Read the model definition and answer for the solid it produces. Units are mm, in the model's axes. Face numbers are marked on the shaded views. A direction names the side the tool comes from. Coordinates: 2 decimals unless noted, no trailing zeros. Write each loop counter-clockwise with the first axis right and the second up, starting at its lowest first coordinate (ties: lowest second). Pieces come first, ordered by that corner, then holes. Notation, with made-up numbers: M 80.5,-20 L 98.5,-20 A26 cw 98.5,0 Z; hole C -24.5,65 d9. An arc over 180 degrees is marked long. Use a Markdown table: item, result. Add a question column.
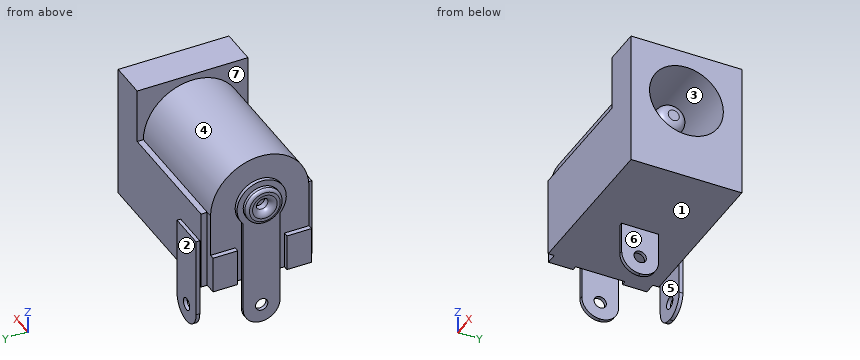
from build123d import *

# Parameters (mm, degrees)
BOSS_EXTRUDE1_DEPTH  = 6.5
BOSS_EXTRUDE2_REACH  = 18.078
SKETCH2_R            = 4
BOSS_EXTRUDE3_DEPTH  = 3
CUT_EXTRUDE1_START   = -0.4
CUT_EXTRUDE1_DEPTH   = 0.4
SKETCH5_W            = 3
SKETCH5_H            = 4
BOSS_EXTRUDE4_DEPTH  = 0.3
SKETCH6_W            = 3
SKETCH6_H            = 0.3
BOSS_EXTRUDE5_DEPTH  = 4
SKETCH7_R            = 0.5
CUT_EXTRUDE4_DEPTH   = 17.01530518
SKETCH8_W            = 6.5
SKETCH8_H            = 0.5
BOSS_EXTRUDE6_DEPTH  = 0.2
BOSS_EXTRUDE7_DEPTH  = 0.3
SKETCH10_W           = 0.3
SKETCH10_H           = 3
BOSS_EXTRUDE8_DEPTH  = 4
SKETCH12_W           = 0.3
SKETCH12_H           = 3
BOSS_EXTRUDE9_DEPTH  = 4
SKETCH11_R           = 0.5
CUT_EXTRUDE5_DEPTH   = 19.364367672
SKETCH13_R           = 3
CUT_EXTRUDE6_DEPTH   = 10
SKETCH14_R           = 1.5
BOSS_EXTRUDE10_DEPTH = 0.5
SKETCH15_R           = 0.5
CUT_EXTRUDE7_DEPTH   = 1
FILLET1_R            = 0.5
FILLET2_R            = 0.25
SKETCH16_R           = 1.2
BOSS_EXTRUDE11_DEPTH = 8
FILLET4_R            = 0.75


with BuildPart() as part:
    # Sketch1 → Boss-Extrude1 (new body)
    with BuildSketch(Plane.XY):
        Polygon((7, 4.5), (-5.873443246, 4.5), (-5.873443246, 4), (-7, 4), (-7, -4), (-5.873443246, -4), (-5.873443246, -4.5), (7, -4.5), align=None)
    extrude(amount=BOSS_EXTRUDE1_DEPTH)

    # Boss-Extrude2: up to this face of the body (flat: up to its plane)
    boss_extrude2_end = Plane(part.part.faces().sort_by_distance((-7, 0, 3.25))[0])
    # Sketch2 → Boss-Extrude2 (add, up to the picked face)
    with BuildSketch(Plane(origin=(7, 0, 0), x_dir=(0, 0, -1), z_dir=(1, 0, 0)), mode=Mode.PRIVATE) as boss_extrude2_sk1:
        with Locations((-6.5, 0)):
            Circle(SKETCH2_R)
    boss_extrude2_tool1 = split(extrude(boss_extrude2_sk1.sketch, amount=-BOSS_EXTRUDE2_REACH, mode=Mode.PRIVATE), bisect_by=boss_extrude2_end, keep=Keep.BOTH, mode=Mode.PRIVATE)
    add(boss_extrude2_tool1.solids().sort_by(Axis((7, 0, 6.5), (-1, 0, 0)))[0])

    # Sketch3 → Boss-Extrude3 (add)
    with BuildSketch(Plane(origin=(7, 0, 0), x_dir=(0, 0, -1), z_dir=(1, 0, 0))):
        with BuildLine():
            Line((-11, -4.5), (-6.5, -4.5))
            Line((-6.5, -4.5), (-6.5, -4))
            ThreePointArc((-6.5, -4), (-10.5, 0), (-6.5, 4))
            Line((-6.5, 4), (-6.5, 4.5))
            Line((-6.5, 4.5), (-11, 4.5))
            Line((-11, 4.5), (-11, 0.782604766))
            Line((-11, 0.782604766), (-11, -4.5))
        make_face()
    extrude(amount=-BOSS_EXTRUDE3_DEPTH)

    # Sketch4 → Cut-Extrude1 (cut)
    with BuildSketch(Plane.ZY.offset(7).offset(CUT_EXTRUDE1_START)):
        with BuildLine():
            Line((3, 4), (3, 2))
            Line((3, 2), (0, 2))
            Line((0, 2), (0, -2))
            Line((0, -2), (3, -2))
            Line((3, -2), (3, -4))
            Line((3, -4), (6.5, -4))
            ThreePointArc((6.5, -4), (10.5, 0), (6.5, 4))
            Line((6.5, 4), (3, 4))
        make_face()
    extrude(amount=CUT_EXTRUDE1_DEPTH, mode=Mode.SUBTRACT)

    # Sketch5 → Boss-Extrude4 (add)
    with BuildSketch(Plane(origin=(0, 4.5, 0), x_dir=(1, 0, 0), z_dir=(0, 1, 0))):
        with Locations((-4.373443246, -2)):
            Rectangle(SKETCH5_W, SKETCH5_H)
    extrude(amount=BOSS_EXTRUDE4_DEPTH)

    # Sketch6 → Boss-Extrude5 (add)
    with BuildSketch(Plane(origin=(0, 0, 0), x_dir=(-1, 0, 0), z_dir=(0, 0, -1))):
        with Locations((4.373443246, 4.65)):
            Rectangle(SKETCH6_W, SKETCH6_H)
    extrude(amount=BOSS_EXTRUDE5_DEPTH)

    # Sketch7 → Cut-Extrude4 (cut, through all)
    with BuildSketch(Plane(origin=(0, 4.8, 0), x_dir=(1, 0, 0), z_dir=(0, 1, 0))):
        with Locations(Location((-4.373443246, 2.5, 0), (0, 0, 270))):
            Circle(SKETCH7_R)
        with BuildLine():
            Line((-5.873443246, 4), (-5.873443246, 2.5))
            ThreePointArc((-5.873443246, 2.5), (-5.434103418, 3.560660172), (-4.373443246, 4))
            Line((-4.373443246, 4), (-5.873443246, 4))
        make_face()
        with BuildLine():
            Line((-2.873443246, 4), (-4.373443246, 4))
            ThreePointArc((-4.373443246, 4), (-3.312783074, 3.560660172), (-2.873443246, 2.5))
            Line((-2.873443246, 2.5), (-2.873443246, 4))
        make_face()
    extrude(amount=-CUT_EXTRUDE4_DEPTH, mode=Mode.SUBTRACT)

    # Sketch8 → Boss-Extrude6 (add)
    with BuildSketch(Plane.ZY.offset(5.873443246)):
        with Locations((3.25, 4.25)):
            Rectangle(SKETCH8_W, SKETCH8_H)
        with Locations((3.25, -4.25)):
            Rectangle(SKETCH8_W, SKETCH8_H)
    extrude(amount=BOSS_EXTRUDE6_DEPTH)

    # Sketch9 → Boss-Extrude7 (add)
    with BuildSketch(Plane.ZY.offset(6.6)):
        with BuildLine():
            Line((5.177124344, 1.5), (0, 1.5))
            Line((0, 1.5), (0, -1.5))
            Line((0, -1.5), (5.177124344, -1.5))
            ThreePointArc((5.177124344, -1.5), (8.5, 0), (5.177124344, 1.5))
        make_face()
    extrude(amount=BOSS_EXTRUDE7_DEPTH)

    # Sketch10 → Boss-Extrude8 (add)
    with BuildSketch(Plane(origin=(0, 0, 0), x_dir=(-1, 0, 0), z_dir=(0, 0, -1))):
        with Locations((6.75, 0)):
            Rectangle(SKETCH10_W, SKETCH10_H)
    extrude(amount=BOSS_EXTRUDE8_DEPTH)

    # Sketch12 → Boss-Extrude9 (add)
    with BuildSketch(Plane(origin=(0, 0, 0), x_dir=(-1, 0, 0), z_dir=(0, 0, -1))):
        with Locations((0.45, 0)):
            Rectangle(SKETCH12_W, SKETCH12_H)
    extrude(amount=BOSS_EXTRUDE9_DEPTH)

    # Sketch11 → Cut-Extrude5 (cut, through all)
    with BuildSketch(Plane.ZY.offset(6.9)):
        with Locations(Location((-2.5, 0, 0), (0, 0, 270))):
            Circle(SKETCH11_R)
        with BuildLine():
            Line((-2.5, 1.5), (-4, 1.5))
            Line((-4, 1.5), (-4, 0))
            ThreePointArc((-4, 0), (-3.560660172, 1.060660172), (-2.5, 1.5))
        make_face()
        with BuildLine():
            ThreePointArc((-2.5, -1.5), (-3.560660172, -1.060660172), (-4, 0))
            Line((-4, 0), (-4, -1.5))
            Line((-4, -1.5), (-2.5, -1.5))
        make_face()
    extrude(amount=-CUT_EXTRUDE5_DEPTH, mode=Mode.SUBTRACT)

    # Sketch13 → Cut-Extrude6 (cut)
    with BuildSketch(Plane(origin=(7, 0, 0), x_dir=(0, 0, -1), z_dir=(1, 0, 0))):
        with Locations(Location((-6.7, 0, 0), (0, 0, 90))):
            Circle(SKETCH13_R)
    extrude(amount=-CUT_EXTRUDE6_DEPTH, mode=Mode.SUBTRACT)

    # Sketch14 → Boss-Extrude10 (add)
    with BuildSketch(Plane.ZY.offset(6.9)):
        with Locations((6.5, 0)):
            Circle(SKETCH14_R)
    extrude(amount=BOSS_EXTRUDE10_DEPTH)

    # Sketch15 → Cut-Extrude7 (cut)
    with BuildSketch(Plane.ZY.offset(7.4)):
        with Locations((6.5, 0)):
            Circle(SKETCH15_R)
    extrude(amount=-CUT_EXTRUDE7_DEPTH, mode=Mode.SUBTRACT)

    # Fillet1
    fillet1_edges = [part.edges().sort_by_distance(p)[0] for p in [
        (-7.4, 0, 6),
    ]]
    fillet(fillet1_edges, radius=FILLET1_R)

    # Fillet2
    fillet2_edges = [part.edges().sort_by_distance(p)[0] for p in [
        (-7.4, 0, 5),
    ]]
    fillet(fillet2_edges, radius=FILLET2_R)

    # Sketch16 → Boss-Extrude11 (add)
    with BuildSketch(Plane(origin=(-3, 0, 0), x_dir=(0, 0, -1), z_dir=(1, 0, 0))):
        with Locations(Location((-6.7, 0, 0), (0, 0, 90))):
            Circle(SKETCH16_R)
    extrude(amount=BOSS_EXTRUDE11_DEPTH)

    # Fillet4
    fillet4_edges = [part.edges().sort_by_distance(p)[0] for p in [
        (5, -1.2, 6.7),
    ]]
    fillet(fillet4_edges, radius=FILLET4_R)


solid = part.part
Item 1: Consider probe 1 along Z at (x, y) = (4.75, 0.25); probe 2 along Z at (x, y) = (-2.5, -0.5); probe 3 along X at (y, z) = (4.7, -2.5). Determine where each line is inside the solid, lowest interval first.
Item 2: Determine the mould class of the marked faces 1, 2, 3 and 4 for opening direction Z: pulls with the +Z half, pulls with the -Z half, needs draft (parallel to the pull), parting line crosses it, or undercut.
Item 3: For the marked faces 5, 6 and 7, determine the directions among +Z, -Z, +X, -X, +Y, -Y from which every point of the face is accessible in a straight line to the end or side of a thin tool.
Item 4: Find section B-B on z = -1.25. Give the vertices of the cut face in (x, y).
Item 5: Each of these flat-tipped pins is pushed along its axis until it touches: pin 1 (0.5 mm diameter, centred on x = -6.5, z = 2.5, fed in from +Y); pin 2 (2.5 mm diameter, centred on y = -0.5, z = -2.5, fed in from +X); pin 3 (3 mm diameter, centred on y = -2, z = 1, fed in from -X). Where does it stop, or does it pass through?
Item 6: Find section A-A on x = -2. Give the vertices of the cut face in (y, z).
Item 7: Find section C-C on z = 1.5. Give the vertices of the cut face in (x, y).
Item 8: Find section D-D on y = 3.5. Give the vertices of the cut face in (x, z).
Geometry says:
| question | item | result |
|---|---|---|
| 1 | probe 1 | z = 0 to 3.71, 5.72 to 7.68, 9.69 to 11 |
| 1 | probe 2 | z = 0 to 3.74, 5.61 to 7.79, 9.66 to 10.47 |
| 1 | probe 3 | x = -5.87 to -4.87, -3.87 to -2.87 |
| 2 | face 1 | pulls with the -Z half |
| 2 | face 2 | needs draft |
| 2 | face 3 | undercut |
| 2 | face 4 | pulls with the +Z half |
| 3 | face 5 | -Z, +X, -X, -Y |
| 3 | face 6 | -Z, +X, +Y, -Y |
| 3 | face 7 | +Z, -X |
| 4 | outline | M -6.9,-1.5 L -6.6,-1.5 L -6.6,1.5 L -6.9,1.5 Z; M -5.87,4.5 L -2.87,4.5 L -2.87,4.8 L -5.87,4.8 Z; M -0.6,-1.5 L -0.3,-1.5 L -0.3,1.5 L -0.6,1.5 Z |
| 5 | pin 1 | stops at y = 4 |
| 5 | pin 2 | stops at x = -0.3 |
| 5 | pin 3 | stops at x = -7 |
| 6 | outline | M -4.5,0 L 4.5,0 L 4.5,6.5 L 4,6.5 A4 ccw -4,6.5 L -4.5,6.5 Z; C 0,6.7 d2.4; hole C 0,6.7 d6 |
| 7 | outline | M -7,-4 L -6.07,-4 L -6.07,-4.5 L 7,-4.5 L 7,4.5 L -2.87,4.5 L -2.87,4.8 L -5.87,4.8 L -5.87,4.5 L -6.07,4.5 L -6.07,4 L -7,4 L -7,2 L -6.6,2 L -6.6,1.5 L -6.9,1.5 L -6.9,-1.5 L -6.6,-1.5 L -6.6,-2 L -7,-2 Z |
| 8 | outline | M -7,0 L 7,0 L 7,11 L 4,11 L 4,8.44 L -6.6,8.44 L -6.6,3 L -7,3 Z |
